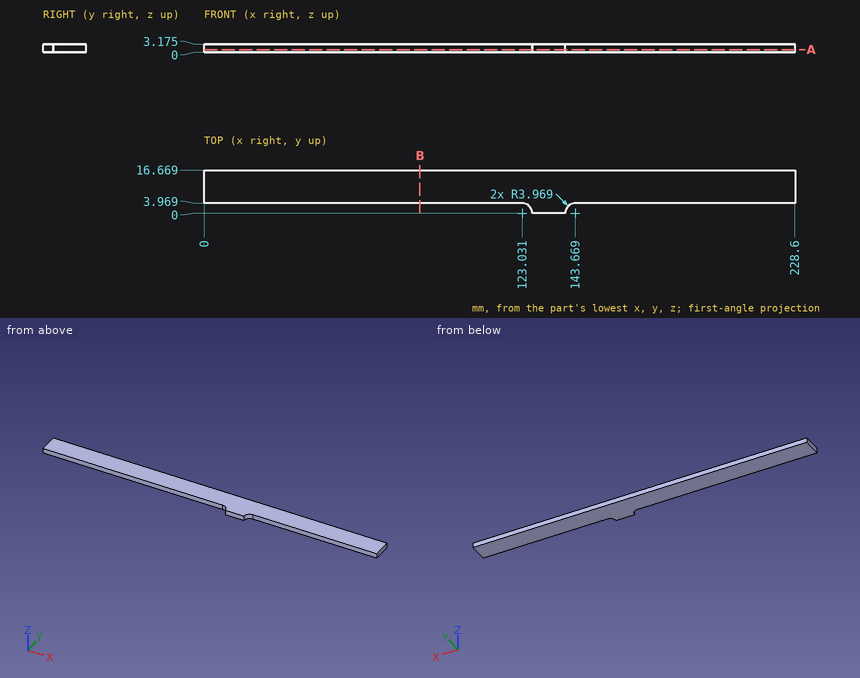
Design review of the part shown in the three views and the two pictorial views. Dimensions are in mm from the part's minimum x, y and z. Round coordinates to 2 decimals unless told otherwise and drop trailing zeros. Write each loop counter-clockwise with the first axis right and the second up, starting at its lowest first coordinate (ties: lowest second). Pieces come first, ordered by that corner, then holes.
Item 1: Consider section B-B on x = 83.5. Give the boundary of the cut face in (y, z) (1 decimal).
Item 2: Consider section A-A on z = 0.95. Give the boundary of the cut face in (x, y).
Item 3: Wall thickness on L1, parallel to Y at x = 51, z = 1.55; L2, parallel to X at y = 2.75, z = 2.5 (1 decimal); L3, parallel to X at y = 2, z = 0.8: over which ranges is each line inside the solid? List them lowest first.
Check values:
1. outline: (4, 0) - (16.7, 0) - (16.7, 3.2) - (4, 3.2) - close
2. outline: (0, 3.97) - (123.03, 3.97) arc R3.97 cw to (127, 0) - (139.7, 0) arc R3.97 cw to (143.67, 3.97) - (228.6, 3.97) - (228.6, 16.67) - (0, 16.67) - close
3. L1: y = 3.97 to 16.67
3. L2: x = 125.9 to 140.8
3. L3: x = 126.46 to 140.24
